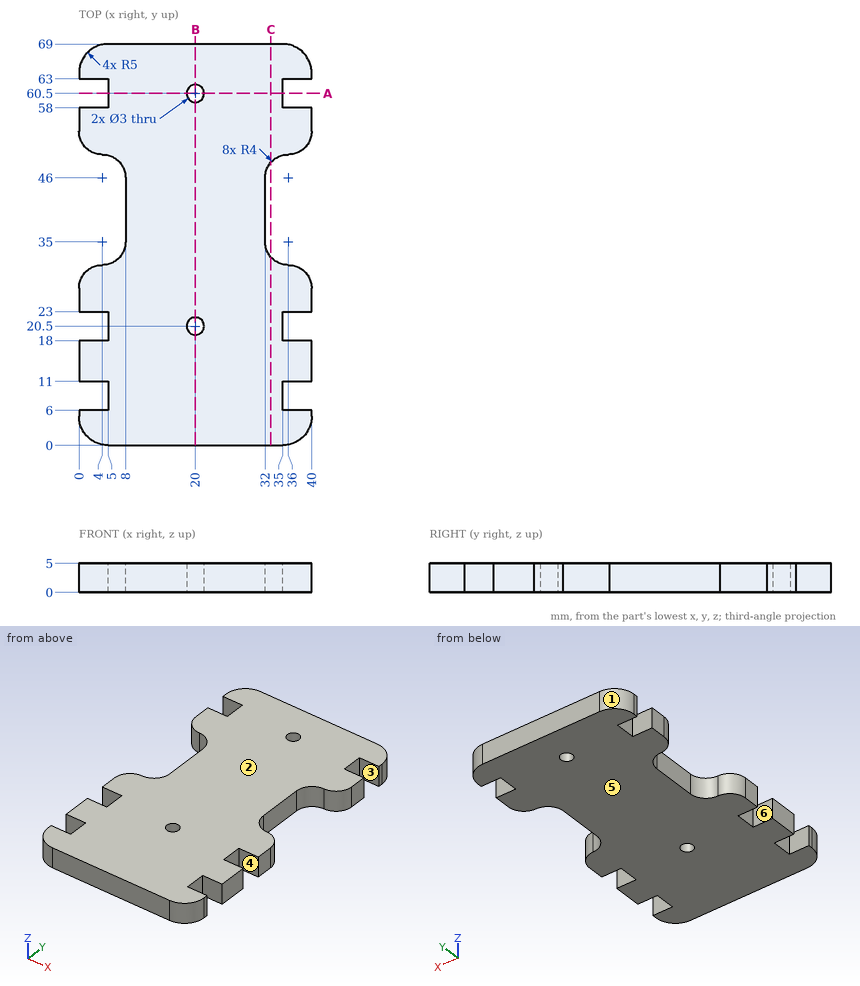
Can you work these out from the drawing? Everything is in mm from the part's minimum corner. A direction names the side the tool comes from. Coordinates: 2 decimals unless noted, no trailing zeros. Write each loop counter-clockwise with the first axis right and the second up, starting at its lowest first coordinate (ties: lowest second). Pieces come first, ordered by that corner, then holes. Notation, with made-up numbers: (-37, 48) -> (-5, 48) arc R20 cw to (-5, 59) -> close; hole circle Ø9 at (-16.5, -23). An arc over 180 degrees is marked (long way). Write each question's results on one line, items separated by ' | '. Start each with the question number.
Item 1: I'm going to push flat-ended pins straight in: P1, Ø1.5, axis at x = 36.5, z = 3.5, coming from the +Y side; P2, Ø1.5, axis at x = 3, z = 3.5, coming from the +Y side; P3, Ø2.5, axis at x = 38, z = 3, coming from the -Y side; P4, Ø2.5, axis at x = 20, y = 20.5, coming from the -Z side. Where does each tip first touch, or does it pass through?
Item 2: If we section it at B-B, the plane x = 20: Write out the boundary of the cut face in (y, z), and give its area (3 significant figures).
Item 3: If we section it at C-C, the plane x = 33: Write out the boundary of the cut face in (y, z), and give its area (3 significant figures).
Item 4: If we section it at A-A, the plane y = 60.5: Write out the boundary of the cut face in (x, z).
Item 5: Thinking about a two-plate mould opening in Y: for the marked faces 1, 2 and 3, which applies, released by +Y, released by -Y, zero draft, split by the parting line, or undercut?
Item 6: Please list where these lines run through material, in increasing order: probe 1 along Y at (x, z) = (20, 2.3); probe 2 along X at (y, z) = (37.5, 2.6); probe 3 along Y at (x, z) = (36.5, 3.1).
Item 7: On a 3-axis mill with a long thin cutter (end or side, diameter ignored), from which of +Z, -Z, +X, -X, +Y, -Y can I reach the whole of each face in a straight line? I mean the marked faces 4, 5 and 6. Say none if no direction works.
Answer block:
1) P1: y = 68.94 | P2: y = 68.84 | P3: y = 0.32 | P4: through
2) outline: (0, 0) -> (19, 0) -> (19, 5) -> (0, 5) -> close; (22, 0) -> (59, 0) -> (59, 5) -> (22, 5) -> close; (62, 0) -> (69, 0) -> (69, 5) -> (62, 5) -> close | area: 315 mm²
3) outline: (0, 0) -> (32.35, 0) -> (32.35, 5) -> (0, 5) -> close; (48.65, 0) -> (69, 0) -> (69, 5) -> (48.65, 5) -> close | area: 264 mm²
4) outline: (5, 0) -> (18.5, 0) -> (18.5, 5) -> (5, 5) -> close; (21.5, 0) -> (35, 0) -> (35, 5) -> (21.5, 5) -> close
5) face 1: released by +Y | face 2: zero draft | face 3: undercut
6) probe 1: 0 to 19, 22 to 59, 62 to 69 | probe 2: 8 to 32 | probe 3: 0.23 to 6, 11 to 18, 23 to 30.97, 50.03 to 58, 63 to 68.77
7) face 4: +Z, -Z, +X | face 5: -Z, +X, -X, +Y, -Y | face 6: +Z, -Z, -X
